Geometry check sheet. Reference: the model listing, model coordinates, mm. A direction names the side the tool comes from. Round coordinates to 2 decimals unless told otherwise and drop trailing zeros. Order: outer loops, then holes, each group sorted by start corner. A loop starts at its lowest first (then second) coordinate and runs counter-clockwise, first axis right, second up. Notation, with made-up numbers: (-24.5, -9) - (30.5, -9) arc R18 cw to (30.5, 22) - close; hole circle Ø9 at (56.5, 75). An arc over 180 degrees is marked (long way). Return JSON: item names as keys, results as strings. Group by question number.
Q1. Tool access check on faces 1 (the flat face through (45, 10, 131)), 2 (the flat face through (35, 85, 140)), 3 (the flat face through (5, 60, 145)), 4 (the flat face through (85, 65, 150)). Record the directions out of +Z, -Z, +X, -X, +Y, -Y that give a thin tool (end or side, any length) a straight path to the whole face; none if there is none.
Q2. Sectioned sample at D-D, the plane y = 7. Record the cut outline in (x, z), then the cut area to 3 significant figures.
Q3. Sectioned sample at B-B, the plane y = 42. Record the cut outline in (x, z).
Q4. Sectioned sample at A-A, the plane z = 120. Record the cut outline in (x, y), then the cut area to 3 significant figures.
Q5. Material ranges on line 1 along X through (y, z) = (12.5, 137); line 2 along Z through (x, y) = (75, 33); line 3 along Z through (x, y) = (8.5, 12), recorded low to high.
Q6. Gauge pin test, flat end, axial feed: pin 1 Ø3 at (x, y) = (75, 5.5) entering from +Z. Record the tip position at first contact, or that the pin passes through.
```python
from build123d import *

# Parameters (mm, degrees)
BOX001_W                 = 110
BOX001_H                 = 10
BOX001_DEPTH             = 10
ARRAY001_Y_COUNT         = 4
ARRAY001_Y_PITCH         = 20
ARRAY001_PLACEMENT_ANGLE = 90
BOX_W                    = 110
BOX_H                    = 10
BOX_DEPTH                = 10
ARRAY_Y_COUNT            = 4
ARRAY_Y_PITCH            = 20
BOX003_W                 = 70
BOX003_H                 = 70
BOX003_DEPTH             = 60
BOX002_W                 = 90
BOX002_H                 = 90
BOX002_DEPTH             = 150


with BuildPart() as array001:
    # Box001 → Box001 (new body)
    with BuildSketch(Plane.XY):
        with Locations((55, 5)):
            Rectangle(BOX001_W, BOX001_H)
    extrude(amount=BOX001_DEPTH)

    # Array001 Y: Array001 ×4


with BuildPart() as array001_1:
    add(array001.part)
    with Locations(*[(0, i * ARRAY001_Y_PITCH, 0) for i in range(1, ARRAY001_Y_COUNT)]):
        add(array001.part)


with BuildPart() as array001_2:
    # Array001 placement: moved
    add(array001_1.part.moved(Location((90, -20, 0))).rotate(Axis((90, -20, 0), (0, 0, 1)), ARRAY001_PLACEMENT_ANGLE))


with BuildPart() as fusion:
    # Box → Box (new body)
    with BuildSketch(Plane.XY):
        with Locations((55, 5)):
            Rectangle(BOX_W, BOX_H)
    extrude(amount=BOX_DEPTH)

    # Array Y: Fusion ×4


with BuildPart() as fusion_1:
    add(fusion.part)
    with Locations(*[(0, i * ARRAY_Y_PITCH, 0) for i in range(1, ARRAY_Y_COUNT)]):
        add(fusion.part)

    # Fusion: union Array001
    add(array001_2.part)


with BuildPart() as fusion_2:
    # Fusion placement: moved
    add(fusion_1.part.moved(Location((-10, 10, 140))))


with BuildPart() as cub002:
    # Box003 → Box003 (new body)
    with BuildSketch(Plane(origin=(10, 10, 112), x_dir=(1, 0, 0), z_dir=(0, 0, 1))):
        with Locations((35, 35)):
            Rectangle(BOX003_W, BOX003_H)
    extrude(amount=BOX003_DEPTH)


with BuildPart() as obj1:
    # Box002 → Box002 (new body)
    with BuildSketch(Plane.XY):
        with Locations((45, 45)):
            Rectangle(BOX002_W, BOX002_H)
    extrude(amount=BOX002_DEPTH)

    # Cut: cut Cub002
    add(cub002.part, mode=Mode.SUBTRACT)

    # Cut001: cut Fusion
    add(fusion_2.part, mode=Mode.SUBTRACT)


solid = obj1.part
```
Reply:
{
 "1": {"face 1": "+Z", "face 2": "+Z, +Y, -Y", "face 3": "+Z, +X, -X", "face 4": "+Z, +X, -X, +Y, -Y"},
 "2": {"outline": "(0, 0) - (90, 0) - (90, 150) - (80, 150) - (80, 140) - (70, 140) - (70, 150) - (60, 150) - (60, 140) - (50, 140) - (50, 150) - (40, 150) - (40, 140) - (30, 140) - (30, 150) - (20, 150) - (20, 140) - (10, 140) - (10, 150) - (0, 150) - close", "area": "13,100 mm^2"},
 "3": {"outline": "(0, 0) - (90, 0) - (90, 150) - (80, 150) - (80, 112) - (10, 112) - (10, 150) - (0, 150) - close"},
 "4": {"outline": "(0, 0) - (90, 0) - (90, 90) - (0, 90) - close; hole (10, 10) - (80, 10) - (80, 80) - (10, 80) - close", "area": "3,200 mm^2"},
 "5": {"line 1": "0 to 10, 80 to 90", "line 2": "0 to 112", "line 3": "0 to 140"},
 "6": {"pin 1": "z = 140"}
}
